Build history of the part. All positions in model axes, mm. Face numbers are marked on the shaded views. Round coordinates to 2 decimals unless told otherwise and drop trailing zeros. Loops run counter-clockwise (first coordinate to the right, second up) from the corner with the lowest first, then second, coordinate; pieces in that order, holes last. Notation, with made-up numbers: (77, 77) - (99, 77) arc R15 cw to (99, 93) - close; hole circle Ø3 at (51, -13.75). An arc over 180 degrees is marked (long way). Use a Markdown table: item, result.
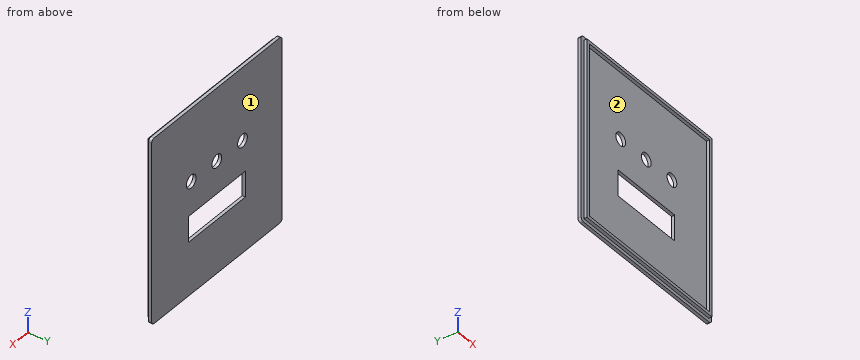
from build123d import *

# Parameters (mm, degrees)
SKETCH1_W           = 157.7
SKETCH1_H           = 169.84
SKETCH1_W_2         = 151.7
SKETCH1_H_2         = 163.84
BOSS_EXTRUDE1_DEPTH = 3
SKETCH2_W           = 164.3
SKETCH2_H           = 176.44
BOSS_EXTRUDE2_DEPTH = 3
SKETCH3_R           = 6.155
SKETCH3_W           = 71.73
SKETCH3_H           = 24.68
CUT_EXTRUDE1_DEPTH  = 3
FILLET1_R           = 3


with BuildPart() as part:
    # Sketch1 → Boss-Extrude1 (new body)
    with BuildSketch(Plane(origin=(0, 0, 0), x_dir=(1, 0, 0), z_dir=(0, 1, 0))):
        Rectangle(SKETCH1_W, SKETCH1_H)
        Rectangle(SKETCH1_W_2, SKETCH1_H_2, mode=Mode.SUBTRACT)
    extrude(amount=BOSS_EXTRUDE1_DEPTH)

    # Sketch2 → Boss-Extrude2 (add)
    with BuildSketch(Plane(origin=(0, 3, 0), x_dir=(1, 0, 0), z_dir=(0, 1, 0))):
        Rectangle(SKETCH2_W, SKETCH2_H)
    extrude(amount=BOSS_EXTRUDE2_DEPTH)

    # Sketch3 → Cut-Extrude1 (cut)
    with BuildSketch(Plane(origin=(0, 6, 0), x_dir=(1, 0, 0), z_dir=(0, 1, 0))):
        with Locations((0, -18.655)):
            Circle(SKETCH3_R)
        with Locations((32.31, -18.655)):
            Circle(SKETCH3_R)
        with Locations((-32.31, -18.655)):
            Circle(SKETCH3_R)
        with Locations((0, 24.84)):
            Rectangle(SKETCH3_W, SKETCH3_H)
    extrude(amount=-CUT_EXTRUDE1_DEPTH, mode=Mode.SUBTRACT)

    # Fillet1
    fillet1_edges = [part.edges().sort_by_distance(p)[0] for p in [
        (82.15, 4.5, 88.22),
        (82.15, 4.5, -88.22),
        (-82.15, 4.5, -88.22),
        (-82.15, 4.5, 88.22),
    ]]
    fillet(fillet1_edges, radius=FILLET1_R)


solid = part.part
Q1. Cut at B-B, the plane x = -8.5. List the corners of the cut face in (y, z).
Results found:
| item | result |
|---|---|
| outline | (0, -84.92) - (3, -84.92) - (3, -88.22) - (6, -88.22) - (6, -37.18) - (3, -37.18) - (3, -81.92) - (0, -81.92) - close; (0, 81.92) - (3, 81.92) - (3, -12.5) - (6, -12.5) - (6, 88.22) - (3, 88.22) - (3, 84.92) - (0, 84.92) - close |
Q2. Cut at C-C, the plane z = -20.5. List the corners of the cut face in (x, y) (3 decimals), plus the area to 3 significant figures.
Results found:
| item | result |
|---|---|
| outline | (-82.15, 3) - (-78.85, 3) - (-78.85, 0) - (-75.85, 0) - (-75.85, 3) - (-35.865, 3) - (-35.865, 6) - (-82.15, 6) - close; (35.865, 3) - (75.85, 3) - (75.85, 0) - (78.85, 0) - (78.85, 3) - (82.15, 3) - (82.15, 6) - (35.865, 6) - close |
| area | 296 mm2 |
Q3. Cut at D-D, the plane y = 1.1. List the corners of the cut face in (x, z).
Results found:
| item | result |
|---|---|
| outline | (-78.85, -84.92) - (78.85, -84.92) - (78.85, 84.92) - (-78.85, 84.92) - close; hole (-75.85, -81.92) - (75.85, -81.92) - (75.85, 81.92) - (-75.85, 81.92) - close |
Q4. Drop flat-ended pins along their axis: pin 1 (1.5 mm diameter, centred on x = -9, y = 2, fed in from +Z); pin 2 (0.9 mm diameter, centred on y = 1.5, z = 26.5, fed in from -X). Give the stop position or say it passes through.
Results found:
| item | result |
|---|---|
| pin 1 | stops at z = 84.92 |
| pin 2 | stops at x = -78.85 |
Q5. Probe line 1 (Z direction, x = -33, y = 5.5); line 2 (X direction, y = 1.5, z = -33); line 3 (Z direction, x = 57, y = 2.5). List the from-to ranges inside material, lowest first.
Results found:
| item | result |
|---|---|
| line 1 | z = -88.22 to -37.18, -12.5 to 12.54, 24.77 to 88.22 |
| line 2 | x = -78.85 to -75.85, 75.85 to 78.85 |
| line 3 | z = -84.92 to -81.92, 81.92 to 84.92 |
Q6. Cut at A-A, the plane x = 32.31. List the corners of the cut face in (y, z), plus the area to 3 significant figures.
Results found:
| item | result |
|---|---|
| outline | (0, -84.92) - (3, -84.92) - (3, -88.22) - (6, -88.22) - (6, -37.18) - (3, -37.18) - (3, -81.92) - (0, -81.92) - close; (0, 81.92) - (3, 81.92) - (3, 24.81) - (6, 24.81) - (6, 88.22) - (3, 88.22) - (3, 84.92) - (0, 84.92) - close; (3, -12.5) - (6, -12.5) - (6, 12.5) - (3, 12.5) - close |
| area | 436 mm2 |
Q7. Pull direction X, two halves, no side cores. Call the marked faces 1 and 2: pulls with the +X half, pulls with the -X half, needs draft (parallel to the pull), parting line crosses it, or undercut.
Results found:
| item | result |
|---|---|
| face 1 | needs draft |
| face 2 | undercut |
